from build123d import *

# Parameters (mm, degrees)
F2_R          = 3.302
F3_DEPTH      = 77.216
F5_START      = -40.64
F4_R          = 3.175
F5_DEPTH      = 60.961
F6_R          = 1.1938
F7_DEPTH      = 25.4
F7_DEPTH_BACK = 25.4


# Not quite as in the source:
# - a feature names something its author has since deleted; it is built from what else it names


with BuildPart() as f1:
    # F0 (on Right) → F1 (revolve)
    with BuildSketch(Plane.YZ):
        with BuildLine():
            Line((0, 12.7), (0, 0))
            Line((0, 0), (101.6, 0))
            Line((101.6, 0), (101.6, 11.8551712597))
            Line((101.6, 11.8551712597), (95.25, 11.8551712597))
            Line((95.25, 11.8551712597), (95.25, 9.0634808418))
            ThreePointArc((95.25, 9.0634808418), (94.1293552402, 6.9632371008), (91.7608131807, 6.7247481879))
            Line((91.7608131807, 6.7247481879), (77.216, 12.7))
            Line((77.216, 12.7), (0, 12.7))
        make_face()
    revolve(axis=Axis((0, 50.8, 0), (0, 1, 0)))

    # F2 (on Front) → F3 (cut)
    with BuildSketch(Plane.XZ):
        with Locations((12.7568459138, 0)):
            Circle(F2_R)
        with Locations((6.3784229569, 11.0477526335)):
            Circle(F2_R)
        with Locations((-6.3784229569, 11.0477526335)):
            Circle(F2_R)
        with Locations((-12.7568459138, 0)):
            Circle(F2_R)
        with Locations((-6.3784229569, -11.0477526335)):
            Circle(F2_R)
        with Locations((6.3784229569, -11.0477526335)):
            Circle(F2_R)
    extrude(amount=-F3_DEPTH, mode=Mode.SUBTRACT)

    # F4 (on Front) → F5 (cut)
    with BuildSketch(Plane.XZ.offset(F5_START)):
        Circle(F4_R)
    extrude(amount=-F5_DEPTH, mode=Mode.SUBTRACT)

    # F6 (on Right) → F7 (cut, two sides)
    with BuildSketch(Plane.YZ) as f7_sk:
        with Locations((67.31, 0)):
            Circle(F6_R)
    extrude(amount=-F7_DEPTH, mode=Mode.SUBTRACT)
    extrude(f7_sk.sketch, amount=F7_DEPTH_BACK, mode=Mode.SUBTRACT)


solid = f1.part
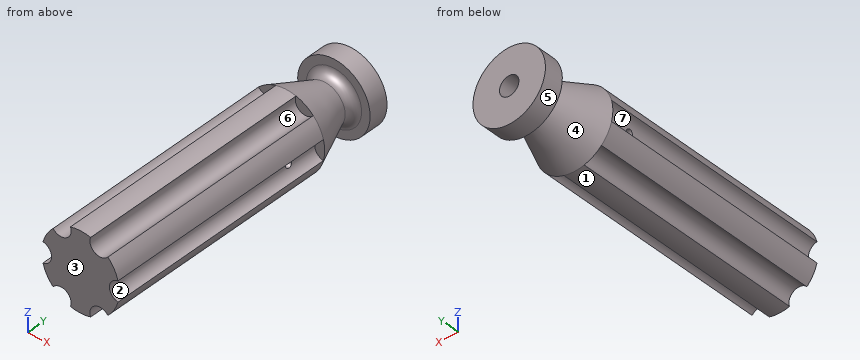
Design review of the part built by this model. Coordinates are the model's own, in mm. Face numbers are marked on the shaded views. A direction names the side the tool comes from. Round coordinates to 2 decimals unless told otherwise and drop trailing zeros. Write each loop counter-clockwise with the first axis right and the second up, starting at its lowest first coordinate (ties: lowest second). Pieces come first, ordered by that corner, then holes. Notation, with made-up numbers: (73.25, 67) - (93.25, 67) arc R27 cw to (93.25, 91) - close; hole circle Ø5 at (56.5, 2.5). An arc over 180 degrees is marked (long way). Return JSON: item names as keys, results as strings. Group by question number.
Item 1: Insertion check: P1, Ø1, axis at x = 9.5, z = -0.5, coming from the -Y side; P2, Ø1.9, axis at x = 0, z = 1.5, coming from the +Y side; P3, Ø3.5, axis at x = -5.5, z = -10, coming from the -Y side; P4, Ø3, axis at y = 42, z = 1, coming from the +X side. Each pin has a flat end and moves straight along its axis. Give the tip position at first contact, or say it passes through.
Item 2: We need section D-D on x = 0. Write out the cut boundary in (y, z) (3 decimals).
Item 3: We need section B-B on y = 38.5. Write out the cut boundary in (x, z).
Item 4: We need section A-A on y = 67.31. Write out the cut boundary in (x, z) (3 decimals), and give its area (3 significant figures).
Item 5: For probe 1 along Z at (x, y) = (0, 69) (3 decimals); probe 2 along Y at (x, z) = (5.25, 0); probe 3 along X at (y, z) = (44.5, 8), list the stretches that pass through material, from the lowest coordinate up. Write a range as [from, to].
Item 6: Machinability: for the marked faces 4, 5, 6 and 7, which of the approach directions +Z, -Z, +X, -X, +Y, -Y give a long, thin tool a straight path to every point of the face, cutting with its end or side? Answer none if there is none.
Item 7: The part is to be moulded in two halves that separate along Z. For the marked faces 1, 2 and 3, say which applies: pulls with the +Z half, pulls with the -Z half, needs draft (parallel to the pull), parting line crosses it, or undercut.
Item 8: We need section C-C on x = 7.5. Give the number of separate pieces and of enclosed holes in the cut face, and give its area (3 significant figures).
Model answer:
{
 "1": {"P1": "stops at y = 0", "P2": "stops at y = 40.64", "P3": "stops at y = 77.22", "P4": "stops at x = 10.6"},
 "2": {"outline": "(0, -12.7) - (77.216, -12.7) - (91.761, -6.725) arc R2.528 cw to (95.25, -9.063) - (95.25, -11.855) - (101.6, -11.855) - (101.6, -3.175) - (40.64, -3.175) - (40.64, 3.175) - (101.6, 3.175) - (101.6, 11.855) - (95.25, 11.855) - (95.25, 9.063) arc R2.528 cw to (91.761, 6.725) - (77.216, 12.7) - (0, 12.7) - close"},
 "3": {"outline": "(-12.27, -3.27) arc R12.7 ccw to (-8.97, -9) arc R3.3 cw to (-3.31, -12.26) arc R12.7 ccw to (3.31, -12.26) arc R3.3 cw to (8.97, -9) arc R12.7 ccw to (12.27, -3.27) arc R3.3 cw to (12.27, 3.27) arc R12.7 ccw to (8.97, 9) arc R3.3 cw to (3.31, 12.26) arc R12.7 ccw to (-3.31, 12.26) arc R3.3 cw to (-8.97, 9) arc R12.7 ccw to (-12.27, 3.27) arc R3.3 cw to start"},
 "4": {"outline": "(-12.273, -3.266) arc R12.7 ccw to (-8.965, -8.995) arc R3.302 cw to (-3.308, -12.262) arc R12.7 ccw to (3.308, -12.262) arc R3.302 cw to (8.965, -8.995) arc R12.7 ccw to (12.273, -3.266) arc R3.302 cw to (9.678, -1.194) - (2.942, -1.194) arc R3.175 cw to (-2.942, -1.194) - (-9.678, -1.194) arc R3.302 cw to start; (-12.273, 3.266) arc R3.302 cw to (-9.678, 1.194) - (-2.942, 1.194) arc R3.175 cw to (2.942, 1.194) - (9.678, 1.194) arc R3.302 cw to (12.273, 3.266) arc R12.7 ccw to (8.965, 8.995) arc R3.302 cw to (3.308, 12.262) arc R12.7 ccw to (-3.308, 12.262) arc R3.302 cw to (-8.965, 8.995) arc R12.7 ccw to start", "area": "349 mm²"},
 "5": {"probe 1": "z = [-12.7, -3.175], [3.175, 12.7]", "probe 2": "y = [0, 66.12], [68.5, 101.6]", "probe 3": "x = [-9.86, -7.65], [-5.11, 5.11], [7.65, 9.86]"},
 "6": {"face 4": "none", "face 5": "+Y", "face 6": "-Y", "face 7": "-X, -Y"},
 "7": {"face 1": "pulls with the -Z half", "face 2": "undercut", "face 3": "needs draft"},
 "8": {"separate pieces": "2", "enclosed holes": "1", "area": "1,510 mm²"}
}
